Autodesk Inventor part; units mm, degrees
ref_plane "YZ Plane" through (0, 0, 0) normal (1, 0, 0) x (0, 1, 0)
ref_plane "XZ Plane" through (0, 0, 0) normal (0, 1, 0) x (-1, 0, 0)
ref_plane "XY Plane" through (0, 0, 0) normal (0, 0, 1) x (1, 0, 0)
sketch "Sketch1" plane through (0, 0, 0) normal (0, 0, 1) x (1, 0, 0)
  arc A0 (0, 16.053) -> (0, -16.053) centre (0, 0) ccw
  arc A1 (-15.7355, 27.991) -> (-17.0055, 26.721) centre (-15.7355, 26.721) ccw
  line L0 (-17.0055, 26.721) -> (-17.0055, 23.52)
  line L1 (-17.0055, 23.52) -> (-18.1469, 23.52)
  line L2 (0, 78.3044) -> (0, -31.8793)
  line L3 (-15.7355, 27.991) -> (0, 27.991)
  line L4 (-18.1469, 23.52) -> (-23.75, 17.9169)
  line L5 (-23.75, 17.9169) -> (-23.75, 14.428)
  line L6 (-23.75, 14.428) -> (-22.174, 12.852)
  line L7 (-22.6105, 9.8935) -> (-21.4771, 9.8935)
  arc A2 (-21.4771, 6.8205) -> (-21.4771, 9.8935) centre (-20.015, 8.357) ccw
  line L8 (-22.942, 6.8205) -> (-21.4771, 6.8205)
  arc A3 (-22.174, 12.852) -> (-22.6105, 9.8935) centre (54.6936, 0) ccw
  arc A4 (-21.544, -9.8935) -> (-21.544, -6.8205) centre (-20.015, -8.357) ccw
  line L9 (-22.942, -6.8205) -> (-21.544, -6.8205)
  line L10 (-22.6105, -9.8935) -> (-21.544, -9.8935)
  arc A5 (-22.942, 6.8205) -> (-22.942, -6.8205) centre (54.6936, 0) ccw
  arc A6 (-22.6105, -9.8935) -> (-22.174, -12.852) centre (54.6936, 0) ccw
  line L11 (-22.174, -12.852) -> (-23.75, -14.428)
  line L12 (-23.75, -14.428) -> (-23.75, -18.4059)
  line L13 (-23.75, -18.4059) -> (-18.1469, -24.009)
  line L14 (-18.1469, -24.009) -> (-14.687, -24.009)
  line L15 (-14.687, -24.009) -> (-12.852, -22.174)
  arc A7 (-6.8205, -21.4771) -> (-9.8935, -21.4771) centre (-8.357, -20.015) ccw
  line L16 (-9.8935, -21.4771) -> (-9.8935, -22.6105)
  line L17 (-6.8205, -21.4771) -> (-6.8205, -22.942)
  arc A8 (-12.852, -22.174) -> (-9.8935, -22.6105) centre (0, 54.6936) ccw
  arc A9 (-6.8205, -22.942) -> (0, -23.241) centre (0, 54.6936) ccw
  circle A10 centre (-17, -17) radius 3
  circle A11 centre (-17, 17) radius 3
  arc A12 (0, -16.053) -> (0, 16.053) centre (0, 0) ccw
  arc A13 (17.0055, 26.721) -> (15.7355, 27.991) centre (15.7355, 26.721) ccw
  line L18 (17.0055, 26.721) -> (17.0055, 23.52)
  line L19 (17.0055, 23.52) -> (18.1469, 23.52)
  line L20 (15.7355, 27.991) -> (0, 27.991)
  line L21 (18.1469, 23.52) -> (23.75, 17.9169)
  line L22 (23.75, 17.9169) -> (23.75, 14.428)
  line L23 (23.75, 14.428) -> (22.174, 12.852)
  line L24 (22.6105, 9.8935) -> (21.4771, 9.8935)
  arc A14 (21.4771, 9.8935) -> (21.4771, 6.8205) centre (20.015, 8.357) ccw
  line L25 (22.942, 6.8205) -> (21.4771, 6.8205)
  arc A15 (22.6105, 9.8935) -> (22.174, 12.852) centre (-54.6936, 0) ccw
  arc A16 (21.544, -6.8205) -> (21.544, -9.8935) centre (20.015, -8.357) ccw
  line L26 (22.942, -6.8205) -> (21.544, -6.8205)
  line L27 (22.6105, -9.8935) -> (21.544, -9.8935)
  arc A17 (22.942, -6.8205) -> (22.942, 6.8205) centre (-54.6936, 0) ccw
  arc A18 (22.174, -12.852) -> (22.6105, -9.8935) centre (-54.6936, 0) ccw
  line L28 (22.174, -12.852) -> (23.75, -14.428)
  line L29 (23.75, -14.428) -> (23.75, -18.4059)
  line L30 (23.75, -18.4059) -> (18.1469, -24.009)
  line L31 (18.1469, -24.009) -> (14.687, -24.009)
  line L32 (14.687, -24.009) -> (12.852, -22.174)
  arc A19 (9.8935, -21.4771) -> (6.8205, -21.4771) centre (8.357, -20.015) ccw
  line L33 (9.8935, -21.4771) -> (9.8935, -22.6105)
  line L34 (6.8205, -21.4771) -> (6.8205, -22.942)
  arc A20 (9.8935, -22.6105) -> (12.852, -22.174) centre (0, 54.6936) ccw
  arc A21 (0, -23.241) -> (6.8205, -22.942) centre (0, 54.6936) ccw
  circle A22 centre (17, -17) radius 3
  circle A23 centre (17, 17) radius 3
  arc A24 (22.174, -12.852) -> (22.6105, -9.8935) centre (-54.6936, 0) ccw
  arc A25 (22.942, -6.8205) -> (22.942, 6.8205) centre (-54.6936, 0) ccw
  dimension "d0" = 54.6936
  dimension "d2" = 54.6936
  dimension "d6" = 32.106
  dimension "d8" = 2.54
  dimension "d10" = 15.7355
  dimension "d11" = 26.721
  dimension "d12" = 18.1469
  dimension "d13" = 23.52
  dimension "d14" = 135
  dimension "d15" = 17.9169
  dimension "d16" = 3.4889
  dimension "d17" = 135
  dimension "d18" = 22.174
  dimension "d19" = 9.8935
  dimension "d22" = 22.6105
  dimension "d23" = 20.015
  dimension "d24" = 8.357
  dimension "d25" = 4.242
  dimension "d26" = 6.8205
  dimension "d27" = 8.357
  dimension "d28" = 4.3354
  dimension "d29" = 6.8205
  dimension "d30" = 9.8935
  dimension "d31" = 77.9346
  dimension "d32" = 22.174
  dimension "d33" = 12.852
  dimension "d34" = 45
  dimension "d35" = 14.428
  dimension "d37" = 18.4059
  dimension "d38" = 135
  dimension "d39" = 24.009
  dimension "d41" = 135
  dimension "d42" = 14.687
  dimension "d43" = 20.015
  dimension "d44" = 8.357
  dimension "d45" = 4.242
  dimension "d46" = 9.8935
  dimension "d47" = 6.8205
  dimension "d48" = 77.9346
  dimension "d49" = 77.9346
  dimension "d50" = 17
  dimension "d51" = 17
  dimension "d52" = 6
  dimension "d53" = 17
  dimension "d54" = 6
extrude "PHD, 32MM" add sketch "Sketch1" against normal blind 25.4 contours A0 L2 A9 L17 A7 L16 A8 L15 L14 L13 L12 L11 A6 L10 A4 L9 A5 L8 A2 L7 A3 L6 L5 L4 L1 L0 A1 L3 | L2 L20 A13 L18 L19 L21 L22 L23 A15 L24 A14 L25 A17 L26 A16 L27 A18 L28 L29 L30 L31 L32 A20 L33 A19 L34 A21 A12
equation "\"d29\" = d26"
equation "\"d54\" = d52"
properties part number "EXTRUSION, CYLINDER, ALUMINIUM, PHD, 32MM" material "Extrusion, Aluminum, PHD, 32MM"
Design review of the part built by this model. Coordinates are the model's own, in mm. A direction names the side the tool comes from. Round coordinates to 2 decimals unless told otherwise and drop trailing zeros. Loops run counter-clockwise (first coordinate to the right, second up) from the corner with the lowest first, then second, coordinate; pieces in that order, holes last. Notation, with made-up numbers: (39.25, 65.5) - (64.25, 65.5) arc R18 cw to (64.25, 83.5) - close; hole circle Ø2 at (9.5, 7.5). An arc over 180 degrees is marked (long way). One line per item, written item: value. Start each with the question number.
1) Consider section B-B on x = -5.5. Give the boundary of the cut face in (y, z).
2) Consider section C-C on y = -17. Give the boundary of the cut face in (x, z), then the cut area to 3 significant figures.
3) For faces 1 (the cylindrical face through (-11.396, -22.403, -12.522)), 2 (the flat face through (-17.006, 25, -13)), 3 (the cylindrical face through (-22.403, 11.396, -12.522)), 4 (the cylindrical face through (22.403, -11.396, -12.522)), list the 3-axis set-ups (+Z, -Z, +X, -X, +Y, -Y) from which the entire face can be reached by the end or side of a thin tool; tool diameter is ignored.
4) To check wall thickness, follow L1, parallel to X at y = -17.5, z = -9.5; L2, parallel to Y at x = 21, z = -5; L3, parallel to X at y = 18, z = -10.25. State the ranges of each line that lie inside material, in increasing order. Write a range as from..to.
5) Consider section A-A on y = 8.5. Give the boundary of the cut face in (x, z).
6) Draft analysis for pull direction Y (two halves, no side actions). For faces 5 (the flat face through (-23.75, 16, -13)), 6 (the cylindrical face through (-16.62, 27.63, -12.52)), 7 (the cylindrical face through (-17.85, -8.43, -12.52)), state which applies: +Y half, -Y half, draft (parallel to the pull), parting line (faces both ways), or undercut.
7) Insertion check: pin 1 Ø2 at (x, z) = (-11, -9.5) entering from -Y; pin 2 Ø6 at (x, y) = (-15, 11.5) entering from +Z; pin 3 Ø1.5 at (y, z) = (2, -15.5) entering from -X; pin 4 Ø0.7 at (y, z) = (-22.5, -15) entering from +X. Each pin has a flat end and moves straight along its axis. Give the tip position at first contact, or say it passes through.
8) Consider section D-D on z = -22.25. Give the number of separate pieces and of enclosed holes in the cut face, then the cut area to 3 significant figures.
Reported:
1. outline: (-23.05, -25.4) - (-15.08, -25.4) - (-15.08, 0) - (-23.05, 0) - close; (15.08, -25.4) - (27.99, -25.4) - (27.99, 0) - (15.08, 0) - close
2. outline: (-23.75, -25.4) - (-20, -25.4) - (-20, 0) - (-23.75, 0) - close; (-14, -25.4) - (14, -25.4) - (14, 0) - (-14, 0) - close; (20, -25.4) - (23.75, -25.4) - (23.75, 0) - (20, 0) - close
2. area: 902 mm^2
3. face 1: +Z, -Z, -Y
3. face 2: +Z, -Z, -X, +Y
3. face 3: +Z, -Z, -X
3. face 4: +Z, -Z, +X
4. L1: x = -23.75..-19.96, -14.04..14.04, 19.96..23.75
4. L2: y = -21.16..-10.29, -6.43..6.48, 10.24..20.67
4. L3: x = -23.67..-19.83, -14.17..14.17, 19.83..23.67
5. outline: (-17.9, -25.4) - (-13.62, -25.4) - (-13.62, 0) - (-17.9, 0) - close; (13.62, -25.4) - (17.9, -25.4) - (17.9, 0) - (13.62, 0) - close
6. face 5: draft
6. face 6: +Y half
6. face 7: undercut
7. pin 1: stops at y = -22.6
7. pin 2: stops at z = 0
7. pin 3: stops at x = -23.23
7. pin 4: stops at x = 20.01
8. separate pieces: 1
8. enclosed holes: 5
8. area: 1,240 mm^2
